The model under review builds one solid part; all positions refer to its coordinate system, in mm. A direction names the side the tool comes from. Coordinates: 2 decimals unless noted, no trailing zeros. Loops run counter-clockwise (first coordinate to the right, second up) from the corner with the lowest first, then second, coordinate; pieces in that order, holes last. Notation, with made-up numbers: M 37.5,68 L 72.5,68 A13 cw 72.5,81 Z; hole C -25,-24.75 d8. An arc over 180 degrees is marked long. One line per item, written item: value.
```python
from build123d import *

# Parameters (mm, degrees)
SKETCH_1_R          = 96.5
EXTRUDE_1_DEPTH     = 45
SKETCH_2_R          = 48.25
CUT_EXTRUDE_1_DEPTH = 42.3
SKETCH_3_W          = 83.620488478
SKETCH_3_H          = 30
CUT_EXTRUDE_2_DEPTH = 500
SKETCH_5_R          = 20
EXTRUDE_2_DEPTH     = 7
SKETCH_8_R          = 1.75
CUT_EXTRUDE_3_DEPTH = 143.876835071


with BuildPart() as part:
    # 草图1 → 凸台-拉伸1 (new body)
    with BuildSketch(Plane(origin=(0, 0, 0), x_dir=(1, 0, 0), z_dir=(0, 1, 0))):
        with Locations(Location((0, 0, 0), (0, 0, 90))):
            Circle(SKETCH_1_R)
    extrude(amount=EXTRUDE_1_DEPTH)

    # 草图2 → 切除-拉伸1 (cut)
    with BuildSketch(Plane(origin=(0, 0, 0), x_dir=(-1, 0, 0), z_dir=(0, -1, 0))):
        with Locations(Location((0, 0, 0), (0, 0, 90))):
            Circle(SKETCH_2_R)
    extrude(amount=-CUT_EXTRUDE_1_DEPTH, mode=Mode.SUBTRACT)

    # 草图3 → 切除-拉伸2 (cut, symmetric)
    with BuildSketch(Plane(origin=(0, 0, 0), x_dir=(0, 0, -1), z_dir=(1, 0, 0))):
        with Locations((0, 23.651984039)):
            Rectangle(SKETCH_3_W, SKETCH_3_H)
    extrude(amount=CUT_EXTRUDE_2_DEPTH, both=True, mode=Mode.SUBTRACT)

    # 草图5 → 凸台-拉伸2 (add)
    with BuildSketch(Plane(origin=(0, 45, 0), x_dir=(1, 0, 0), z_dir=(0, 1, 0))):
        with Locations(Location((0, 0, 0), (0, 0, 270))):
            Circle(SKETCH_5_R)
    extrude(amount=EXTRUDE_2_DEPTH)

    # 草图8 → 切除-拉伸3 (cut, through all)
    with BuildSketch(Plane(origin=(0, 42.3, 0), x_dir=(-1, 0, 0), z_dir=(0, -1, 0))):
        with Locations(Location((0, -44.5, 0), (0, 0, 90))):
            Circle(SKETCH_8_R)
        with Locations(Location((-31.466251763, -31.466251763, 0), (0, 0, 90))):
            Circle(SKETCH_8_R)
        with Locations(Location((-44.5, 0, 0), (0, 0, 90))):
            Circle(SKETCH_8_R)
        with Locations(Location((-31.466251763, 31.466251763, 0), (0, 0, 90))):
            Circle(SKETCH_8_R)
        with Locations(Location((0, 44.5, 0), (0, 0, 90))):
            Circle(SKETCH_8_R)
        with Locations(Location((31.466251763, 31.466251763, 0), (0, 0, 90))):
            Circle(SKETCH_8_R)
        with Locations(Location((44.5, 0, 0), (0, 0, 90))):
            Circle(SKETCH_8_R)
        with Locations(Location((31.466251763, -31.466251763, 0), (0, 0, 90))):
            Circle(SKETCH_8_R)
    extrude(amount=-CUT_EXTRUDE_3_DEPTH, mode=Mode.SUBTRACT)


solid = part.part
```
(1) Tool access review of faces 5 (the face through (20.1, 0, 44.2)), 6 (the face through (14.493, 20.854, -46.022)), 7 (the face through (69, 8.652, 1)): name each direction out of +Z, -Z, +X, -X, +Y, -Y from which nothing blocks a thin tool from reaching the whole face with its end or side.
Checks:
face 5: +Z, -Z, +X, -X, -Y
face 6: -Y
face 7: +X, -X
(2) Add section C-C on x = -77.5. State the section outline as (y, z) points, then the cut area to 3 significant figures.
Checks:
outline: M 0,-57.5 L 45,-57.5 L 45,57.5 L 0,57.5 Z; hole M 8.65,-41.81 L 38.65,-41.81 L 38.65,41.81 L 8.65,41.81 Z
area: 2,670 mm^2
(3) To check wall thickness, follow L1, parallel to Y at x = -31, z = -39.5; L2, parallel to X at y = 43.75, z = -44.5; L3, parallel to Y at x = 54.5, z = 60.5. State the ranges of each line that lie inside material, in increasing order. Write a range as [from, to].
Checks:
L1: [0, 8.65], [38.65, 45]
L2: [-85.63, -1.75], [1.75, 85.63]
L3: [0, 45]
(4) Add section A-A on y = 27. State the section outline as (x, z) points, then the cut area to 3 significant figures.
Checks:
outline: M -86.97,-41.81 A96.5 ccw 86.97,-41.81 L 24.08,-41.81 A48.25 cw -24.08,-41.81 Z; M -86.97,41.81 L -24.08,41.81 A48.25 cw 24.08,41.81 L 86.97,41.81 A96.5 ccw Z
area: 13,200 mm^2
(5) Add section B-B on z = 5. State the section outline as (x, y) points.
Checks:
outline: M -96.37,0 L -47.99,0 L -47.99,8.65 L -96.37,8.65 Z; M -96.37,38.65 L -47.99,38.65 L -47.99,42.3 L 47.99,42.3 L 47.99,38.65 L 96.37,38.65 L 96.37,45 L 19.36,45 L 19.36,52 L -19.36,52 L -19.36,45 L -96.37,45 Z; M 47.99,0 L 96.37,0 L 96.37,8.65 L 47.99,8.65 Z
(6) Add section D-D on x = 39.5. State the section outline as (y, z) points, then the cut area to 3 significant figures.
Checks:
outline: M 0,-88.05 L 45,-88.05 L 45,88.05 L 0,88.05 L 0,27.71 L 8.65,27.71 L 8.65,41.81 L 38.65,41.81 L 38.65,27.71 L 42.3,27.71 L 42.3,-27.71 L 38.65,-27.71 L 38.65,-41.81 L 8.65,-41.81 L 8.65,-27.71 L 0,-27.71 Z
area: 4,730 mm^2
(7) Insertion check: pin 1 Ø12 at (y, z) = (41.5, 48) entering from +X; pin 2 Ø10 at (x, y) = (-48.5, 22.5) entering from -Z; pin 3 Ø2 at (x, y) = (-25, 43) entering from -Z; pin 4 Ø10 at (y, z) = (40.5, -4) entering from +X. Each pin has a flat end and moves straight along its axis. Give the tip position at first contact, or say it passes through.
Checks:
pin 1: x = 86.88
pin 2: z = -86.14
pin 3: z = -93.47
pin 4: x = 96.5
(8) Draft analysis for pull direction Z (two halves, no side actions). For faces 1 (the face through (69, 38.652, 1)), 2 (the face through (-19.524, 48.451, -4.336)), 3 (the face through (0, 52, 0)), 4 (the face through (1, 42.3, 1)), state which applies: pulls with the +Z half, pulls with the -Z half, needs draft (parallel to the pull), parting line crosses it, or undercut.
Checks:
face 1: undercut
face 2: parting line crosses it
face 3: needs draft
face 4: undercut
